from build123d import *

# Parameters (mm, degrees)
BOSS_EXTRUDE1_DEPTH      = 88.9
CUT_EXTRUDE2_DEPTH       = 241.232341963
CUT_EXTRUDE2_DEPTH_BACK  = 241.232341963
SKETCH3_R                = 28.575
CUT_EXTRUDE5_DEPTH       = 28.575
CUT_EXTRUDE6_DEPTH       = 243.134084755
CUT_EXTRUDE6_DEPTH_BACK  = 243.134084755
SKETCH4_R                = 12.7
CUT_EXTRUDE7_DEPTH       = 261.369359036
CUT_EXTRUDE7_DEPTH_BACK  = 261.369359036
CUT_EXTRUDE8_DEPTH       = 261.369359036
CUT_EXTRUDE8_DEPTH_BACK  = 12.7
SKETCH6_R                = 9.525
SKETCH7_R                = 6.35
CUT_EXTRUDE9_DEPTH       = 12.7
SKETCH12_R               = 12.7
CUT_EXTRUDE13_DEPTH      = 3.175
CUT_EXTRUDE14_DEPTH      = 253.187753717
CUT_EXTRUDE14_DEPTH_BACK = 253.187753717
SKETCH14_R               = 1.5875
CUT_EXTRUDE15_START      = -12.7
CUT_EXTRUDE15_DEPTH      = 12.7
CUT_EXTRUDE16_START      = -12.7
SKETCH8_4_R              = 6.35
CUT_EXTRUDE16_DEPTH      = 19.05
CUT_EXTRUDE18_START      = -171.45
CUT_EXTRUDE18_DEPTH      = 12.7
CUT_EXTRUDE19_START      = -139.7
SKETCH8_10_R             = 6.35
CUT_EXTRUDE19_DEPTH      = 19.05
SKETCH15_R               = 6.35
CUT_EXTRUDE20_DEPTH      = 19.05
CHAMFER1_SIZE            = 2


with BuildPart() as part:
    # Sketch1 → Boss-Extrude1 (new body)
    with BuildSketch(Plane.XY):
        Polygon((0, 0), (0, -174.625), (171.45, -174.625), (171.45, 0), (158.75, 0), (158.75, -142.875), (12.7, -142.875), (12.7, 0), align=None)
    extrude(amount=BOSS_EXTRUDE1_DEPTH)

    # Sketch2 → Cut-Extrude2 (cut, two sides: drawn at the far end of the back side and taken through both)
    with BuildSketch(Plane(origin=(0, -142.875, 0), x_dir=(1, 0, 0), z_dir=(0, 1, 0)).offset(-CUT_EXTRUDE2_DEPTH_BACK)):
        Polygon((158.75, 0), (12.7, 0), (12.7, -25.4), (85.724999876, -25.4), (158.75, -25.4), align=None)
    extrude(amount=CUT_EXTRUDE2_DEPTH + CUT_EXTRUDE2_DEPTH_BACK, mode=Mode.SUBTRACT)

    # Sketch3 → Cut-Extrude5 (cut)
    with BuildSketch(Plane.XZ.offset(174.625)):
        with Locations((85.725, 57.15)):
            Circle(SKETCH3_R)
    extrude(amount=-CUT_EXTRUDE5_DEPTH, mode=Mode.SUBTRACT)

    # Sketch4 → Cut-Extrude6 (cut, two sides: drawn at the far end of the back side and taken through both)
    with BuildSketch(Plane.XZ.offset(146.05).offset(-CUT_EXTRUDE6_DEPTH_BACK)):
        with Locations((85.725, 57.15)):
            Circle(SKETCH4_R)
    extrude(amount=CUT_EXTRUDE6_DEPTH + CUT_EXTRUDE6_DEPTH_BACK, mode=Mode.SUBTRACT)

    # Sketch5 → Cut-Extrude7 (cut, two sides: drawn at the far end of the back side and taken through both)
    with BuildSketch(Plane(origin=(171.45, 0, 0), x_dir=(0, 0, -1), z_dir=(1, 0, 0)).offset(-CUT_EXTRUDE7_DEPTH_BACK)):
        with BuildLine():
            Line((0, -174.625), (0, -114.3))
            ThreePointArc((0, -114.3), (-0.597344099, -119.776153781), (-2.361280333, -124.994736842))
            Line((-2.361280333, -124.994736842), (-25.4, -174.625))
            Line((-25.4, -174.625), (0, -174.625))
        make_face()
        with BuildLine():
            Line((-39.269490456, -98.025866748), (-71.745289975, -22.119448379))
            ThreePointArc((-71.745289975, -22.119448379), (-70.400400796, -7.131859618), (-57.149999966, 0))
            Line((-57.149999966, 0), (-88.9, 0))
            Line((-88.9, 0), (-88.9, -142.875))
            Line((-88.9, -142.875), (-50.8, -142.875))
            Line((-50.8, -142.875), (-39.583234749, -118.711720996))
            ThreePointArc((-39.583234749, -118.711720996), (-37.224875429, -108.402184034), (-39.269490456, -98.025866748))
        make_face()
        with BuildLine():
            Line((0, 0), (-57.149999966, 0))
            ThreePointArc((-57.149999966, 0), (-48.406859618, -2.624599204), (-42.554710025, -9.630551621))
            Line((-42.554710025, -9.630551621), (-2.047536041, -104.308882594))
            ThreePointArc((-2.047536041, -104.308882594), (-0.51714863, -109.200616928), (0, -114.3))
            Line((0, -114.3), (0, 0))
        make_face()
    extrude(amount=CUT_EXTRUDE7_DEPTH + CUT_EXTRUDE7_DEPTH_BACK, mode=Mode.SUBTRACT)

    # Sketch6 → Cut-Extrude8 (cut, two sides: drawn at the far end of the back side and taken through both)
    with BuildSketch(Plane(origin=(171.45, 0, 0), x_dir=(0, 0, -1), z_dir=(1, 0, 0)).offset(-CUT_EXTRUDE8_DEPTH_BACK)):
        with Locations(Location((-57.15, -15.875, 0), (0, 0, 90))):
            Circle(SKETCH6_R)
    extrude(amount=CUT_EXTRUDE8_DEPTH + CUT_EXTRUDE8_DEPTH_BACK, mode=Mode.SUBTRACT)

    # Sketch7 → Cut-Extrude9 (cut)
    with BuildSketch(Plane(origin=(12.7, 0, 0), x_dir=(0, 0, -1), z_dir=(1, 0, 0))):
        with Locations((-57.15, -15.875)):
            Circle(SKETCH7_R)
    extrude(amount=-CUT_EXTRUDE9_DEPTH, mode=Mode.SUBTRACT)

    # Sketch12 → Cut-Extrude13 (cut)
    with BuildSketch(Plane(origin=(12.7, 0, 0), x_dir=(0, 0, -1), z_dir=(1, 0, 0))):
        with Locations((-57.15, -15.875)):
            Circle(SKETCH12_R)
    extrude(amount=-CUT_EXTRUDE13_DEPTH, mode=Mode.SUBTRACT)

    # Sketch14 → Cut-Extrude14 (cut, two sides: drawn at the far end of the back side and taken through both)
    with BuildSketch(Plane(origin=(12.7, 0, 0), x_dir=(0, 0, -1), z_dir=(1, 0, 0)).offset(-CUT_EXTRUDE14_DEPTH_BACK)):
        with Locations((-53.770765225, -24.780413934)):
            Circle(SKETCH14_R)
        with Locations((-66.551932086, -14.348796194)):
            Circle(SKETCH14_R)
        with Locations((-51.12730269, -8.495789872)):
            Circle(SKETCH14_R)
    extrude(amount=CUT_EXTRUDE14_DEPTH + CUT_EXTRUDE14_DEPTH_BACK, mode=Mode.SUBTRACT)

    # Sketch8 → Cut-Extrude15 (cut)
    with BuildSketch(Plane(origin=(171.45, 0, 0), x_dir=(0, 0, -1), z_dir=(1, 0, 0)).offset(CUT_EXTRUDE15_START)):
        with BuildLine():
            Line((-50.8, -142.875), (-88.9, -142.875))
            Line((-88.9, -142.875), (-88.9, -174.625))
            Line((-88.9, -174.625), (-25.4, -174.625))
            Line((-25.4, -174.625), (-2.361280333, -124.994736842))
            ThreePointArc((-2.361280333, -124.994736842), (-0.002921013, -114.68519988), (-2.047536041, -104.308882594))
            Line((-2.047536041, -104.308882594), (-42.554710025, -9.630551621))
            ThreePointArc((-42.554710025, -9.630551621), (-63.394448379, -1.279710025), (-71.745289975, -22.119448379))
            Line((-71.745289975, -22.119448379), (-39.269490456, -98.025866748))
            ThreePointArc((-39.269490456, -98.025866748), (-37.224875429, -108.402184034), (-39.583234749, -118.711720996))
            Line((-39.583234749, -118.711720996), (-50.8, -142.875))
        make_face()
    extrude(amount=CUT_EXTRUDE15_DEPTH, mode=Mode.SUBTRACT)

    # Sketch8<4> → Cut-Extrude16 (cut)
    with BuildSketch(Plane(origin=(171.45, 0, 0), x_dir=(0, 0, -1), z_dir=(1, 0, 0)).offset(CUT_EXTRUDE16_START)):
        with Locations(Location((-76.2, -158.75, 0), (0, 0, 90))):
            Circle(SKETCH8_4_R)
        with Locations(Location((-38.1, -158.75, 0), (0, 0, 90))):
            Circle(SKETCH8_4_R)
    extrude(amount=-CUT_EXTRUDE16_DEPTH, mode=Mode.SUBTRACT)

    # Sketch8<9> → Cut-Extrude18 (cut)
    with BuildSketch(Plane(origin=(171.45, 0, 0), x_dir=(0, 0, -1), z_dir=(1, 0, 0)).offset(CUT_EXTRUDE18_START)):
        with BuildLine():
            Line((-50.8, -142.875), (-88.9, -142.875))
            Line((-88.9, -142.875), (-88.9, -174.625))
            Line((-88.9, -174.625), (-25.4, -174.625))
            Line((-25.4, -174.625), (-2.361280333, -124.994736842))
            ThreePointArc((-2.361280333, -124.994736842), (-0.002921013, -114.68519988), (-2.047536041, -104.308882594))
            Line((-2.047536041, -104.308882594), (-42.554710025, -9.630551621))
            ThreePointArc((-42.554710025, -9.630551621), (-63.394448379, -1.279710025), (-71.745289975, -22.119448379))
            Line((-71.745289975, -22.119448379), (-39.269490456, -98.025866748))
            ThreePointArc((-39.269490456, -98.025866748), (-37.224875429, -108.402184034), (-39.583234749, -118.711720996))
            Line((-39.583234749, -118.711720996), (-50.8, -142.875))
        make_face()
    extrude(amount=CUT_EXTRUDE18_DEPTH, mode=Mode.SUBTRACT)

    # Sketch8<10> → Cut-Extrude19 (cut)
    with BuildSketch(Plane(origin=(171.45, 0, 0), x_dir=(0, 0, -1), z_dir=(1, 0, 0)).offset(CUT_EXTRUDE19_START)):
        with Locations(Location((-76.2, -158.75, 0), (0, 0, 90))):
            Circle(SKETCH8_10_R)
        with Locations(Location((-38.1, -158.75, 0), (0, 0, 90))):
            Circle(SKETCH8_10_R)
    extrude(amount=-CUT_EXTRUDE19_DEPTH, mode=Mode.SUBTRACT)

    # Sketch15 → Cut-Extrude20 (cut)
    with BuildSketch(Plane.XZ.offset(174.625)):
        with Locations((140.97, 73.025)):
            Circle(SKETCH15_R)
        with Locations((140.97, 41.275)):
            Circle(SKETCH15_R)
    extrude(amount=-CUT_EXTRUDE20_DEPTH, mode=Mode.SUBTRACT)

    # Chamfer1
    chamfer1_edges = [part.edges().sort_by_distance(p)[0] for p in [
        (57.15, -174.625, 57.15),
    ]]
    chamfer(chamfer1_edges, length=CHAMFER1_SIZE)


solid = part.part
Can you work these out from the model? Positions are in its coordinate system, mm. A direction names the side the tool comes from. Coordinates: 2 decimals unless noted, no trailing zeros. Loops run counter-clockwise (first coordinate to the right, second up) from the corner with the lowest first, then second, coordinate; pieces in that order, holes last. Notation, with made-up numbers: M 7.5,25.25 L 39.5,25.25 A19 ccw 39.5,41.25 Z; hole C 10.25,72 d7. An arc over 180 degrees is marked long. Return JSON: item names as keys, results as strings. Group by question number.
Item 1: On a 3-axis mill with a long thin cutter (end or side, diameter ignored), from which of +Z, -Z, +X, -X, +Y, -Y can I reach the whole of each face in a straight line? I mean faces 4 (the flat face through (85, -159, 88.9)), 5 (the flat face through (139.7, -156.6, 34.6)), 6 (the cylindrical face through (135.9, -167.4, 69.2)), 7 (the flat face through (31.75, -159, 38)). Say none if no direction works.
Item 2: If I drill on L1, parallel to Y at x = 150.75, z = 76.2 (3 decimals); L2, parallel to X at y = -167, z = 58; L3, parallel to Z at x = 151.25, y = -158.75, over which ranges is the centre line in solid material (lowest first)? Write a range as from..to.
Item 3: Imagine slicing it at C-C (y = -171). Please give me the cut outline in (x, z) (3 decimals), and give its area (3 significant figures).
Item 4: Imagine slicing it at B-B (y = -147.5). Please give me the cut outline in (x, z) (3 decimals), and give its area (3 significant figures).
Item 5: Thinking about a two-plate mould opening in Z: for faces 1 (the cylindrical face through (149.358, -152.884, 35.668)), 2 (the flat face through (12.7, -159, 58)), 3 (the flat face through (85, -159, 25.4)), which applies, released by +Z, released by -Z, zero draft, split by the parting line, or undercut?
Item 6: I'm going to push flat-ended pins straight in: pin 1 Ø6.5 at (y, z) = (-156.5, 74.5) entering from -X; pin 2 Ø3 at (y, z) = (-162.5, 42.5) entering from +X; pin 3 Ø6 at (y, z) = (-158, 36.5) entering from +X; pin 4 Ø7.5 at (x, z) = (140.97, 41.275) entering from -Y (3 decimals). Where does each tip first touch, or does it pass through?
Item 7: Imagine slicing it at D-D (y = -161). Please give me the cut outline in (x, z) (3 decimals).
Item 8: Imagine slicing it at A-A (z = 57.15). Please give me the cut outline in (x, y) (3 decimals), and give its area (3 significant figures).
Verdict:
{
 "1": {"face 4": "+Z, +X, -X, +Y, -Y", "face 5": "+X", "face 6": "-Y", "face 7": "-X"},
 "2": {"L1": "y = -174.625..-165.1, -152.4..-142.875", "L2": "x = 12.7..57.16, 114.29..158.75", "L3": "z = 25.4..31.75, 44.45..69.85, 82.55..88.9"},
 "3": {"outline": "M 12.7,25.4 L 158.75,25.4 L 158.75,88.9 L 12.7,88.9 Z; hole C 85.725,57.15 d57.15; hole C 140.97,41.275 d12.7; hole C 140.97,73.025 d12.7", "area": "6,460 mm^2"},
 "4": {"outline": "M 12.7,25.4 L 158.75,25.4 L 158.75,88.9 L 12.7,88.9 Z; hole C 85.725,57.15 d57.15", "area": "6,710 mm^2"},
 "5": {"face 1": "undercut", "face 2": "zero draft", "face 3": "released by -Z"},
 "6": {"pin 1": "stops at x = 31.75", "pin 2": "stops at x = 158.75", "pin 3": "stops at x = 139.7", "pin 4": "stops at y = -155.575"},
 "7": {"outline": "M 12.7,25.4 L 158.75,25.4 L 158.75,32.162 L 139.7,32.162 L 139.7,35.053 A6.35 cw long 146.687,44.038 L 158.75,44.038 L 158.75,70.262 L 146.687,70.262 A6.35 cw long 139.7,79.247 L 139.7,82.138 L 158.75,82.138 L 158.75,88.9 L 12.7,88.9 L 12.7,82.138 L 31.75,82.138 L 31.75,70.262 L 12.7,70.262 L 12.7,44.038 L 31.75,44.038 L 31.75,32.162 L 12.7,32.162 Z; hole C 85.725,57.15 d57.15"},
 "8": {"outline": "M 12.7,-174.625 L 55.15,-174.625 L 57.15,-172.625 L 57.15,-146.05 L 73.025,-146.05 L 73.025,-142.875 L 12.7,-142.875 Z; M 98.425,-146.05 L 114.3,-146.05 L 114.3,-172.625 L 116.3,-174.625 L 158.75,-174.625 L 158.75,-142.875 L 98.425,-142.875 Z", "area": "2,920 mm^2"}
}
